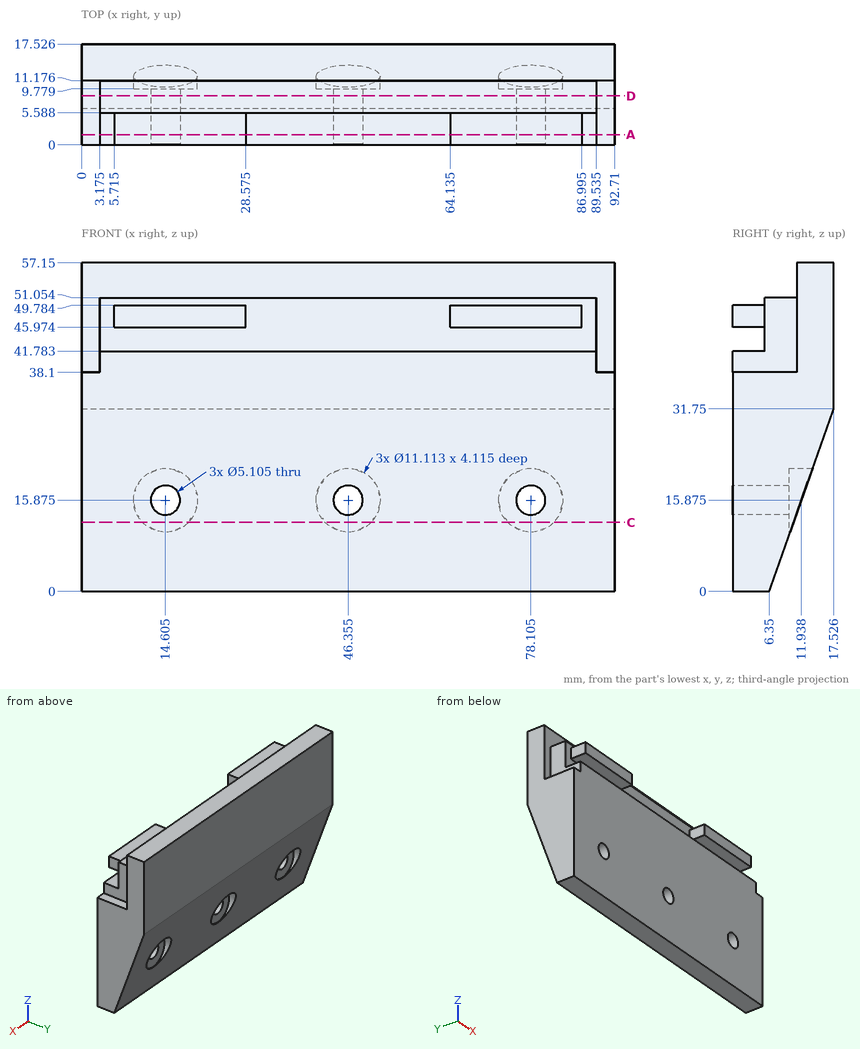
Study the drawing (mm; zero at the part's minimum x, y, z) and answer. Coordinates: 2 decimals unless noted, no trailing zeros. Order: outer loops, then holes, each group sorted by start corner. A loop starts at its lowest first (then second) coordinate and runs counter-clockwise, first axis right, second up. Notation, with made-up numbers: (21, 78) -> (54, 78) arc R12 cw to (54, 87) -> close; hole circle Ø11 at (-34.75, -15). An arc over 180 degrees is marked (long way). Answer in a Markdown table with one row per item. Add a question column.
Item 1: Find the intervals of material crossed by L1, parallel to X at y = 3.5, z = 17 (1 decimal); L2, parallel to Z at x = 6, y = 3.25 (1 decimal); L3, parallel to X at y = 1.25, z = 48.5 (1 decimal), in increasing order. Write a range as from..to.
Item 2: Find section A-A (y = 1.75). Write down the section's boundary in (x, z) (1 decimal), then the cut area to 3 significant figures.
Item 3: Find section C-C (z = 12). Write down the section's boundary in (x, y) (1 decimal).
Item 4: Find section D-D (y = 8.5). Write down the section's boundary in (x, z) (1 decimal).
Item 5: Each of these flat-tipped pins is pushed along its axis until it touches: P1, Ø3.5, axis at x = 44, z = 17, coming from the +Y side; P2, Ø3, axis at y = 2, z = 48.5, coming from the -X side (1 decimal); P3, Ø4, axis at y = 1.5, z = 48.5, coming from the +X side (1 decimal). Where does it stop, or does it pass through?
Result set:
| question | item | result |
|---|---|---|
| 1 | L1 | x = 0..12.3, 16.9..44.1, 48.6..75.8, 80.4..92.7 |
| 1 | L2 | z = 0..41.8, 46..49.8 |
| 1 | L3 | x = 5.7..28.6, 64.1..87 |
| 2 | outline | (0, 0) -> (92.7, 0) -> (92.7, 38.1) -> (89.5, 38.1) -> (89.5, 41.8) -> (3.2, 41.8) -> (3.2, 38.1) -> (0, 38.1) -> close; (5.7, 46) -> (28.6, 46) -> (28.6, 49.8) -> (5.7, 49.8) -> close; (64.1, 46) -> (87, 46) -> (87, 49.8) -> (64.1, 49.8) -> close; hole circle Ø5.1 at (14.6, 15.9); hole circle Ø5.1 at (46.4, 15.9); hole circle Ø5.1 at (78.1, 15.9) |
| 2 | area | 3,960 mm² |
| 3 | outline | (0, 0) -> (92.7, 0) -> (92.7, 10.6) -> (82.1, 10.6) -> (82.1, 9.8) -> (74.1, 9.8) -> (74.1, 10.6) -> (50.3, 10.6) -> (50.3, 9.8) -> (42.4, 9.8) -> (42.4, 10.6) -> (18.6, 10.6) -> (18.6, 9.8) -> (10.6, 9.8) -> (10.6, 10.6) -> (0, 10.6) -> close |
| 4 | outline | (0, 6.1) -> (92.7, 6.1) -> (92.7, 38.1) -> (89.5, 38.1) -> (89.5, 51.1) -> (3.2, 51.1) -> (3.2, 38.1) -> (0, 38.1) -> close; hole circle Ø5.1 at (14.6, 15.9); hole circle Ø5.1 at (46.4, 15.9); hole circle Ø5.1 at (78.1, 15.9) |
| 5 | P1 | stops at y = 9.78 |
| 5 | P2 | stops at x = 5.7 |
| 5 | P3 | stops at x = 87 |
